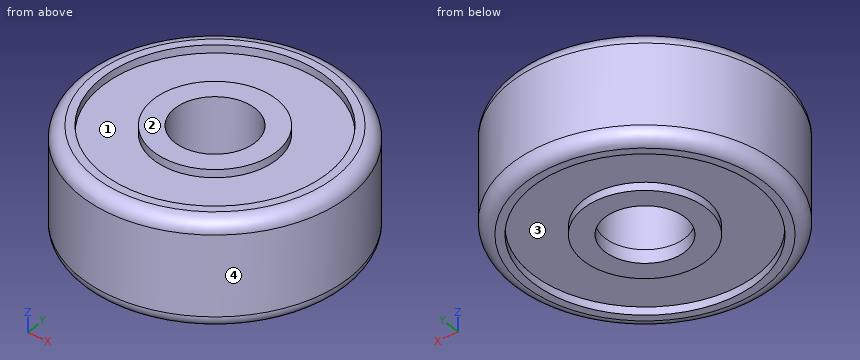
from build123d import *

# Parameters (mm, degrees)
F0_R     = 5
F0_R_2   = 4.2
F1_DEPTH = 3.5
F0_R_3   = 2.3
F2_DEPTH = 3.2
F0_R_4   = 1.5
F3_DEPTH = 3.5
F4_DEPTH = 0.5
F5_DEPTH = 0.5
F6_DEPTH = 0.2
F7_R     = 0.49999


# Not quite as in the source:
# - a fillet or chamfer is up to 0.001 mm smaller than in the source, because OpenCascade refuses the exact size


with BuildPart() as f1:
    # F0 (on Top) → F1 (new body)
    with BuildSketch(Plane.XY):
        Circle(F0_R)
        Circle(F0_R_2, mode=Mode.SUBTRACT)
    extrude(amount=F1_DEPTH)

    # F0 (on Top) → F2 (join)
    with BuildSketch(Plane.XY):
        Circle(F0_R_2)
        Circle(F0_R_3, mode=Mode.SUBTRACT)
    extrude(amount=F2_DEPTH)

    # F0 (on Top) → F3 (join)
    with BuildSketch(Plane.XY):
        Circle(F0_R_3)
        Circle(F0_R_4, mode=Mode.SUBTRACT)
    extrude(amount=F3_DEPTH)

    # F0 (on Top) → F4 (join)
    with BuildSketch(Plane.XY):
        Circle(F0_R)
        Circle(F0_R_2, mode=Mode.SUBTRACT)
    extrude(amount=-F4_DEPTH)

    # F0 (on Top) → F5 (join)
    with BuildSketch(Plane.XY):
        Circle(F0_R_3)
        Circle(F0_R_4, mode=Mode.SUBTRACT)
    extrude(amount=-F5_DEPTH)

    # F0 (on Top) → F6 (join)
    with BuildSketch(Plane.XY):
        Circle(F0_R_2)
        Circle(F0_R_3, mode=Mode.SUBTRACT)
    extrude(amount=-F6_DEPTH)

    # F7 (radius 0.5 in the source; OpenCascade refuses exactly that, so slightly less here)
    f7_edges = [f1.edges().sort_by_distance(p)[0] for p in [
        (-5, 0, 3.5),
        (-5, 0, -0.5),
    ]]
    fillet(f7_edges, radius=F7_R)


solid = f1.part
For this review, take the finished solid that the model builds, in its own axes (mm). Face numbers are marked on the shaded views. Round coordinates to 2 decimals unless told otherwise and drop trailing zeros. Write each loop counter-clockwise with the first axis right and the second up, starting at its lowest first coordinate (ties: lowest second). Pieces come first, ordered by that corner, then holes. Notation, with made-up numbers: (76, 1.25) - (107, 1.25) arc R27 cw to (107, 36.25) - close; hole circle Ø8 at (65, -34). An arc over 180 degrees is marked (long way). Use a Markdown table: item, result.
Q1. The part is to be moulded in two halves that separate along X. For the marked faces 1, 2, 3 and 4, say which applies: pulls with the +X half, pulls with the -X half, needs draft (parallel to the pull), parting line crosses it, or undercut.
Derived:
| item | result |
|---|---|
| face 1 | undercut |
| face 2 | needs draft |
| face 3 | undercut |
| face 4 | parting line crosses it |
Q2. We need section C-C (z = 2.5). Give the boundary of the cut face in (x, y), plus the area to 3 significant figures.
Derived:
| item | result |
|---|---|
| outline | circle Ø10 at (0, 0); hole circle Ø3 at (0, 0) |
| area | 71.5 mm2 |
Q3. Wall thickness on line 1 along X through (y, z) = (0.25, 3.25); line 2 along Y through (x, z) = (0, 3.35); line 3 along Y through (x, z) = (0, 2.55): over which ranges is each line inside the solid? List them lowest first.
Derived:
| item | result |
|---|---|
| line 1 | x = -4.93 to -4.19, -2.29 to -1.48, 1.48 to 2.29, 4.19 to 4.93 |
| line 2 | y = -4.86 to -4.2, -2.3 to -1.5, 1.5 to 2.3, 4.2 to 4.86 |
| line 3 | y = -5 to -1.5, 1.5 to 5 |
Q4. We need section A-A (y = 0). Give the boundary of the cut face in (x, z), plus the area to 3 significant figures.
Derived:
| item | result |
|---|---|
| outline | (-5, 0) arc R0.5 ccw to (-4.5, -0.5) - (-4.2, -0.5) - (-4.2, -0.2) - (-2.3, -0.2) - (-2.3, -0.5) - (-1.5, -0.5) - (-1.5, 3.5) - (-2.3, 3.5) - (-2.3, 3.2) - (-4.2, 3.2) - (-4.2, 3.5) - (-4.5, 3.5) arc R0.5 ccw to (-5, 3) - close; (1.5, -0.5) - (2.3, -0.5) - (2.3, -0.2) - (4.2, -0.2) - (4.2, -0.5) - (4.5, -0.5) arc R0.5 ccw to (5, 0) - (5, 3) arc R0.5 ccw to (4.5, 3.5) - (4.2, 3.5) - (4.2, 3.2) - (2.3, 3.2) - (2.3, 3.5) - (1.5, 3.5) - close |
| area | 25.5 mm2 |
Q5. Clearance check with flat-ended pins moving along their axes: pin 1 (2 mm diameter, centred on x = 2.5, y = -4, fed in from +Z); pin 2 (1.5 mm diameter, centred on y = 4, z = 2.5, fed in from -X). State where each tip first meets the part, or that it passes through.
Derived:
| item | result |
|---|---|
| pin 1 | stops at z = 3.5 |
| pin 2 | stops at x = -3.8 |
